Source: CAD feature listing. Evaluate the final solid. Frame: model axes, mm. Round coordinates to 2 decimals unless told otherwise and drop trailing zeros. Loops run counter-clockwise (first coordinate to the right, second up) from the corner with the lowest first, then second, coordinate; pieces in that order, holes last. Notation, with made-up numbers: M 9.25,1.25 L 68.25,1.25 A22 cw 68.25,15.25 Z; hole C 67.5,65 d8. An arc over 180 degrees is marked long. Answer as a JSON object with one key per item and string values.
from build123d import *

# Parameters (mm, degrees)
SKETCH1_W                   = 130
SKETCH1_H                   = 80
BOSS_EXTRUDE1_DEPTH         = 3
SKETCH2_W                   = 14.444444444
SKETCH2_H                   = 3
SKETCH2_W_2                 = 3
SKETCH2_H_2                 = 13.333333334
SKETCH2_H_3                 = 13.333333333
CUT_EXTRUDE1_DEPTH          = 153.672852859
CUT_CORNERPIECE_HOLES_REACH = 154.673
SKETCH3_R                   = 1.7
CUT_EXTRUDE3_REACH          = 154.673


with BuildPart() as part:
    # Sketch1 → Boss-Extrude1 (new body)
    with BuildSketch(Plane.XY):
        with Locations((65, 40)):
            Rectangle(SKETCH1_W, SKETCH1_H)
    extrude(amount=BOSS_EXTRUDE1_DEPTH)

    # Sketch2 → Cut-Extrude1 (cut, through all)
    with BuildSketch(Plane.XY.offset(3)):
        with Locations((7.222222222, 1.5)):
            Rectangle(SKETCH2_W, SKETCH2_H)
        with Locations((36.111111111, 1.5)):
            Rectangle(SKETCH2_W, SKETCH2_H)
        with Locations((65, 1.5)):
            Rectangle(SKETCH2_W, SKETCH2_H)
        with Locations((93.888888889, 1.5)):
            Rectangle(SKETCH2_W, SKETCH2_H)
        Polygon((115.555555556, 0), (115.555555556, 3), (127, 3), (127, 13.333333333), (130, 13.333333333), (130, 0), align=None)
        with Locations((1.5, 20)):
            Rectangle(SKETCH2_W_2, SKETCH2_H_2)
        with Locations((1.5, 46.666666667)):
            Rectangle(SKETCH2_W_2, SKETCH2_H_3)
        with Locations((1.5, 73.333333334)):
            Rectangle(SKETCH2_W_2, SKETCH2_H_3)
        with Locations((128.5, 33.333333334)):
            Rectangle(SKETCH2_W_2, SKETCH2_H_3)
        with Locations((128.5, 60)):
            Rectangle(SKETCH2_W_2, SKETCH2_H_2)
    extrude(amount=-CUT_EXTRUDE1_DEPTH, mode=Mode.SUBTRACT)

    # Sketch3 → Cut cornerpiece holes (cut, up to next)
    with BuildSketch(Plane.XY.offset(3), mode=Mode.PRIVATE) as cut_cornerpiece_holes_sk1:
        with Locations((15, 74.5)):
            Circle(SKETCH3_R)
    cut_cornerpiece_holes_tool1 = extrude(cut_cornerpiece_holes_sk1.sketch, amount=-CUT_CORNERPIECE_HOLES_REACH, mode=Mode.PRIVATE) & part.part
    # Sketch3 → Cut cornerpiece holes (cut, up to next)
    with BuildSketch(Plane.XY.offset(3), mode=Mode.PRIVATE) as cut_cornerpiece_holes_sk2:
        with Locations((115, 74.5)):
            Circle(SKETCH3_R)
    cut_cornerpiece_holes_tool2 = extrude(cut_cornerpiece_holes_sk2.sketch, amount=-CUT_CORNERPIECE_HOLES_REACH, mode=Mode.PRIVATE) & part.part
    # Sketch3 → Cut cornerpiece holes (cut, up to next)
    with BuildSketch(Plane.XY.offset(3), mode=Mode.PRIVATE) as cut_cornerpiece_holes_sk3:
        with Locations((15, 8.5)):
            Circle(SKETCH3_R)
    cut_cornerpiece_holes_tool3 = extrude(cut_cornerpiece_holes_sk3.sketch, amount=-CUT_CORNERPIECE_HOLES_REACH, mode=Mode.PRIVATE) & part.part
    # Sketch3 → Cut cornerpiece holes (cut, up to next)
    with BuildSketch(Plane.XY.offset(3), mode=Mode.PRIVATE) as cut_cornerpiece_holes_sk4:
        with Locations((115, 8.5)):
            Circle(SKETCH3_R)
    cut_cornerpiece_holes_tool4 = extrude(cut_cornerpiece_holes_sk4.sketch, amount=-CUT_CORNERPIECE_HOLES_REACH, mode=Mode.PRIVATE) & part.part
    add(cut_cornerpiece_holes_tool1.solids().sort_by_distance((15, 74.5, 3))[0], mode=Mode.SUBTRACT)
    add(cut_cornerpiece_holes_tool2.solids().sort_by_distance((115, 74.5, 3))[0], mode=Mode.SUBTRACT)
    add(cut_cornerpiece_holes_tool3.solids().sort_by_distance((15, 8.5, 3))[0], mode=Mode.SUBTRACT)
    add(cut_cornerpiece_holes_tool4.solids().sort_by_distance((115, 8.5, 3))[0], mode=Mode.SUBTRACT)

    # Sketch4 → Cut-Extrude3 (cut, up to next)
    with BuildSketch(Plane(origin=(0, 0, 0), x_dir=(-1, 0, 0), z_dir=(0, 0, -1)), mode=Mode.PRIVATE) as cut_extrude3_sk1:
        with BuildLine():
            Line((-29.825, 55.4), (-20.425, 55.4))
            ThreePointArc((-20.425, 55.4), (-19.358058262, 55.841941738), (-19.8, 54.775))
            Line((-19.8, 54.775), (-19.8, 23.625))
            ThreePointArc((-19.8, 23.625), (-19.358058262, 22.558058262), (-20.425, 23))
            Line((-20.425, 23), (-29.825, 23))
            ThreePointArc((-29.825, 23), (-30.891941738, 22.558058262), (-30.45, 23.625))
            Line((-30.45, 23.625), (-30.45, 54.775))
            ThreePointArc((-30.45, 54.775), (-30.891941738, 55.841941738), (-29.825, 55.4))
        make_face()
    cut_extrude3_tool1 = extrude(cut_extrude3_sk1.sketch, amount=-CUT_EXTRUDE3_REACH, mode=Mode.PRIVATE) & part.part
    add(cut_extrude3_tool1.solids().sort_by_distance((25.125, 39.2, 0))[0], mode=Mode.SUBTRACT)


solid = part.part
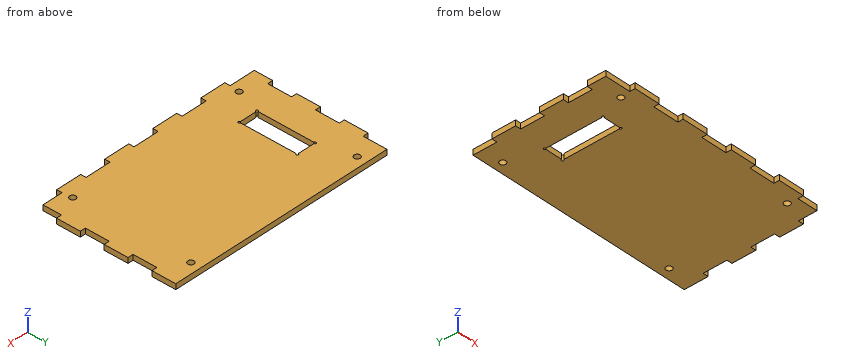
Item 1: Section B-B on y = 74.5. Return the cut outline in (x, z), then the cut area to 3 significant figures.
Answer sheet:
{"outline": "M 3,0 L 13.3,0 L 13.3,3 L 3,3 Z; M 16.7,0 L 113.3,0 L 113.3,3 L 16.7,3 Z; M 116.7,0 L 130,0 L 130,3 L 116.7,3 Z", "area": "361 mm²"}
Item 2: Section C-C on z = 2.15. Give the number of separate pieces and of enclosed holes in the cut face, then the cut area to 3 significant figures.
Answer sheet:
{"separate pieces": "1", "enclosed holes": "5", "area": "9,570 mm²"}
Item 3: Line query: probe 1 along Y at (x, z) = (15, 2.05); probe 2 along X at (y, z) = (74.5, 2.4); probe 3 along X at (y, z) = (7.5, 2.45). Output: solid intervals per line, ascending. Write a range as from..to.
Answer sheet:
{"probe 1": "y = 0..6.8, 10.2..72.8, 76.2..80", "probe 2": "x = 3..13.3, 16.7..113.3, 116.7..130", "probe 3": "x = 0..13.63, 16.37..113.63, 116.37..127"}
Item 4: Section A-A on y = 51.5. Return the cut outline in (x, z).
Answer sheet:
{"outline": "M 3,0 L 19.8,0 L 19.8,3 L 3,3 Z; M 30.45,0 L 130,0 L 130,3 L 30.45,3 Z"}
Item 5: Contact query for flat-ended pins moving along their axis: pin 1 Ø1.5 at (y, z) = (34.5, 1) entering from +X; pin 2 Ø4.5 at (x, y) = (15, 74.5) entering from -Z; pin 3 Ø0.9 at (x, z) = (128.5, 1) entering from -Y; pin 4 Ø1 at (x, y) = (30.45, 23) entering from +Z. Output: stop coordinate, or through.
Answer sheet:
{"pin 1": "stops at x = 127", "pin 2": "stops at z = 0", "pin 3": "stops at y = 13.33", "pin 4": "passes through"}
